Autodesk Inventor part; units mm, degrees
ref_plane "YZ Plane" through (0, 0, 0) normal (1, 0, 0) x (0, 1, 0)
ref_plane "XZ Plane" through (0, 0, 0) normal (0, 1, 0) x (-1, 0, 0)
ref_plane "XY Plane" through (0, 0, 0) normal (0, 0, 1) x (1, 0, 0)
sketch "Sketch1" plane through (0, 0, 0) normal (0, 1, 0) x (-1, 0, 0)
  line L0 (0, 0) -> (19.05, 0)
  line L1 (19.05, 0) -> (19.05, 44.45)
  line L2 (19.05, 44.45) -> (0, 44.45)
  line L3 (0, 44.45) -> (0, 0)
  dimension "d0" = 19.05
  dimension "d1" = 44.45
extrude "Extrusion1" add sketch "Sketch1" along normal blind 25.4
sketch "Sketch2" plane through (0, 0, 44.45) normal (1, 0, 0) x (0, 0, -1)
  line L0 (0, 0) -> (44.45, 0)
  line L1 (0, 0) -> (0, 25.4)
  line L2 (44.45, 0) -> (44.45, 25.4)
  point P0 (6.35, 12.7)
  point P1 (34.925, 12.7)
  point P2 (44.45, 12.7)
  dimension "d4" = 12.7
  dimension "d5" = 12.7
  dimension "d6" = 6.35
  dimension "d7" = 9.525
hole "Hole1" at (0, 12.7, 38.1) direction (-1, 0, 0) diameter 6.5278 depth 50.8 tip angle 118
sketch "Sketch3" plane through (0, 0, 0) normal (0, -1, 0) x (1, 0, 0)
  line L0 (0, 44.45) -> (0, 0)
  line L1 (-19.05, 44.45) -> (0, 44.45)
  point P0 (-9.525, 28.575)
  point P1 (-9.525, 9.6957)
  dimension "d15" = 9.525
  dimension "d16" = 15.875
hole "Hole2" at (-9.525, 0, 28.575) direction (0, 1, 0) diameter 6.5278 depth 50.8 tip angle 118
sketch "Sketch4" plane through (0, 0, 44.45) normal (1, 0, 0) x (0, 0, -1)
  line L0 (0, 25.4) -> (44.45, 25.4)
  line L1 (0, 0) -> (0, 25.4)
  point P0 (44.45, 0)
  point P1 (28.575, 12.7)
  dimension "d24" = 12.7
  dimension "d25" = 28.575
sketch "Sketch5" plane through (0, 0, 0) normal (0, -1, 0) x (1, 0, 0)
  line L0 (0, 44.45) -> (0, 0)
  line L1 (0, 0) -> (-19.05, 0)
  point P0 (-9.525, 6.35)
  dimension "d26" = 9.525
  dimension "d27" = 6.35
hole "Hole3" at (-9.525, 0, 6.35) direction (0, 1, 0) diameter 6.5278 depth 50.8 tip angle 118
hole "Hole4" at (0, 12.7, 15.875) direction (-1, 0, 0) diameter 6.5278 depth 50.8 tip angle 118
properties part number "200522"
For this review, take the finished solid that the model builds, in its own axes (mm). Give positions to 0.01 mm unless a question says otherwise; leave off trailing zeros. Write each loop counter-clockwise with the first axis right and the second up, starting at its lowest first coordinate (ties: lowest second). Pieces come first, ordered by that corner, then holes. Notation, with made-up numbers: (46, 11) -> (89, 11) arc R16 ccw to (89, 16) -> close; hole circle Ø2 at (68.5, 9). An arc over 180 degrees is marked (long way). Use CSV: the item, a comma, the result in double quotes.
Q1. For P1, Ø6, axis at x = -9.5, z = 28, coming from the -Y side, flat-tipped, find the tip position at first contact; note if it passes through.
Conclusion:
P1,"y = 0"
Q2. Take a section at A-A, the plane z = 6.35. Write out the cut boundary in (x, y), then the cut area to 3 significant figures.
Conclusion:
outline,"(-19.05, 0) -> (-12.79, 0) -> (-12.79, 25.4) -> (-19.05, 25.4) -> close; (-6.26, 0) -> (0, 0) -> (0, 25.4) -> (-6.26, 25.4) -> close"
area,"318 mm2"
Q3. Take a section at C-C, the plane x = -15.5. Write out the cut boundary in (y, z) (3 decimals).
Conclusion:
outline,"(0, 0) -> (25.4, 0) -> (25.4, 44.45) -> (0, 44.45) -> close; hole circle Ø6.528 at (12.7, 15.875); hole circle Ø6.528 at (12.7, 38.1)"
Q4. Take a section at B-B, the plane y = 12.7. Write out the cut boundary in (x, z) (3 decimals).
Conclusion:
outline,"(-19.05, 0) -> (0, 0) -> (0, 12.611) -> (-19.05, 12.611) -> close; (-19.05, 19.139) -> (0, 19.139) -> (0, 34.836) -> (-19.05, 34.836) -> close; (-19.05, 41.364) -> (0, 41.364) -> (0, 44.45) -> (-19.05, 44.45) -> close; hole circle Ø6.528 at (-9.525, 6.35); hole circle Ø6.528 at (-9.525, 28.575)"
Q5. Mouldability with a two-part tool opening along Y and no side actions: class faces 1 (the face through (-9.66, 12.56, 41.36)), 2 (the face through (-9, 25.4, 23)), 3 (the face through (-6.63, 12.88, 4.84)) as pulls with the +Y half, pulls with the -Y half, needs draft (parallel to the pull), parting line crosses it, or undercut.
Conclusion:
face 1,"undercut"
face 2,"pulls with the +Y half"
face 3,"needs draft"
Q6. Take a section at D-D, the plane z = 38.1. Write out the cut boundary in (x, y), then the cut area to 3 significant figures.
Conclusion:
outline,"(-19.05, 0) -> (0, 0) -> (0, 9.44) -> (-19.05, 9.44) -> close; (-19.05, 15.96) -> (0, 15.96) -> (0, 25.4) -> (-19.05, 25.4) -> close"
area,"360 mm2"
Q7. To check wall thickness, follow probe 1 along Z at (x, y) = (-8.5, 12); probe 2 along Z at (x, y) = (-9.25, 21.75); probe 3 along Z at (x, y) = (-17.5, 13). State the ranges of each line that lie inside material, in increasing order. Write a range as [from, to].
Conclusion:
probe 1,"[0, 3.25], [9.45, 12.69], [19.06, 25.48], [31.67, 34.91], [41.29, 44.45]"
probe 2,"[0, 3.1], [9.6, 25.32], [31.83, 44.45]"
probe 3,"[0, 12.62], [19.13, 34.85], [41.35, 44.45]"
